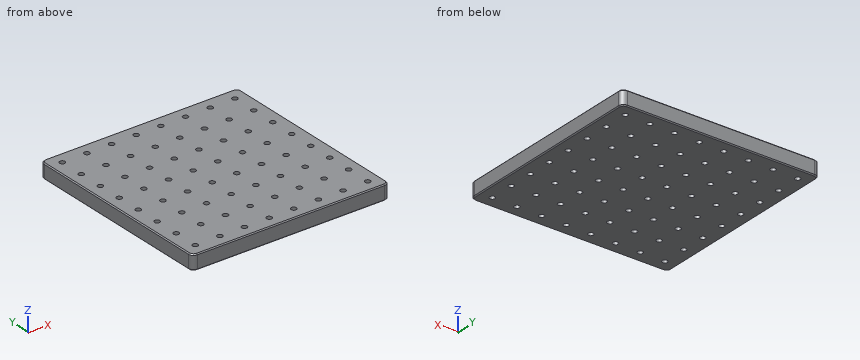
from build123d import *

# Parameters (mm, degrees)
SKETCH1_W            = 400
SKETCH1_H            = 400
BOSS_EXTRUDE1_DEPTH  = 15
LPATTERN1_COUNT      = 8
LPATTERN1_PITCH      = 50
LPATTERN1_COUNT_DIR2 = 8
LPATTERN1_PITCH_DIR2 = 50
FILLET1_R            = 10
CHAMFER1_SIZE        = 2
CHAMFER2_SIZE        = 2


with BuildPart() as part:
    # Sketch1 → Boss-Extrude1 (new body, symmetric)
    with BuildSketch(Plane.XY):
        Rectangle(SKETCH1_W, SKETCH1_H)
    extrude(amount=BOSS_EXTRUDE1_DEPTH, both=True)

    # Sketch2 → M12x1.25 Tapped Hole1 (revolve, cut)
    with BuildSketch(Plane(origin=(-175, 175, 15), x_dir=(0, -1, 0), z_dir=(1, 0, 0))):
        Polygon((0, 0), (0, 33.244647343), (5.4, 30), (5.4, 0), align=None)
    m12x1_25_tapped_hole1 = revolve(axis=Axis((-175, 175, 21.35), (0, 0, -1)), mode=Mode.SUBTRACT)

    # LPattern1: M12x1.25 Tapped Hole1 8 × 8
    with Locations(*[(i * LPATTERN1_PITCH, -j * LPATTERN1_PITCH_DIR2, 0) for i in range(LPATTERN1_COUNT) for j in range(LPATTERN1_COUNT_DIR2) if (i, j) != (0, 0)]):
        add(m12x1_25_tapped_hole1, mode=Mode.SUBTRACT)

    # Fillet1
    fillet1_edges = [part.edges().sort_by_distance(p)[0] for p in [
        (200, -200, 0),
        (-200, -200, 0),
        (-200, 200, 0),
        (200, 200, 0),
    ]]
    fillet(fillet1_edges, radius=FILLET1_R)

    # Chamfer1
    chamfer1_edges = [part.edges().sort_by_distance(p)[0] for p in [
        (200, 0, 15),
        (0, -200, 15),
        (0, 200, 15),
        (-200, 0, 15),
        (-197.071067812, -197.071067812, 15),
        (-197.071067812, 197.071067812, 15),
        (197.071067812, 197.071067812, 15),
        (197.071067812, -197.071067812, 15),
    ]]
    chamfer(chamfer1_edges, length=CHAMFER1_SIZE)

    # Chamfer2
    chamfer2_edges = [part.edges().sort_by_distance(p)[0] for p in [
        (200, 0, -15),
        (0, -200, -15),
        (-200, 0, -15),
        (0, 200, -15),
        (-197.071067812, -197.071067812, -15),
        (-197.071067812, 197.071067812, -15),
        (197.071067812, 197.071067812, -15),
        (197.071067812, -197.071067812, -15),
    ]]
    chamfer(chamfer2_edges, length=CHAMFER2_SIZE)


solid = part.part
The model under review builds one solid part; all positions refer to its coordinate system, in mm. Round coordinates to 2 decimals unless told otherwise and drop trailing zeros. Write item = value, one per line. Start each with the question number.
Item 1: Consider section A-A on x = 25. Count the separate pieces of the cut face and the enclosed holes in it, plus the area to 3 significant figures.
Item 2: Clearance check with a flat-ended pin moving along its axis: pin 1 Ø14 at (x, y) = (175, 125) entering from -Z. State where the tip first meets the part, or that it passes through.
Item 3: For line 1 along Y through (x, z) = (115, -13.5), list the stretches that pass through material, from the lowest coordinate up.
Conclusion:
q1.separate_pieces = 9
q1.enclosed_holes = 0
q1.area = 9,400 mm2
q2.pin_1 = -15
q3.line_1 = -199.5 to 199.5
